The figure shows three views and two pictorial views of one solid part (mm, origin at its lowest corner). Answer the questions. Give positions to 0.01 mm unless a question says otherwise; leave off trailing zeros. Write each loop counter-clockwise with the first axis right and the second up, starting at its lowest first coordinate (ties: lowest second). Pieces come first, ordered by that corner, then holes. Notation, with made-up numbers: (-23, 77) -> (30, 77) arc R27 cw to (30, 106) -> close; hole circle Ø5 at (-11, -29). An arc over 180 degrees is marked (long way). Use a Markdown table: item, result.
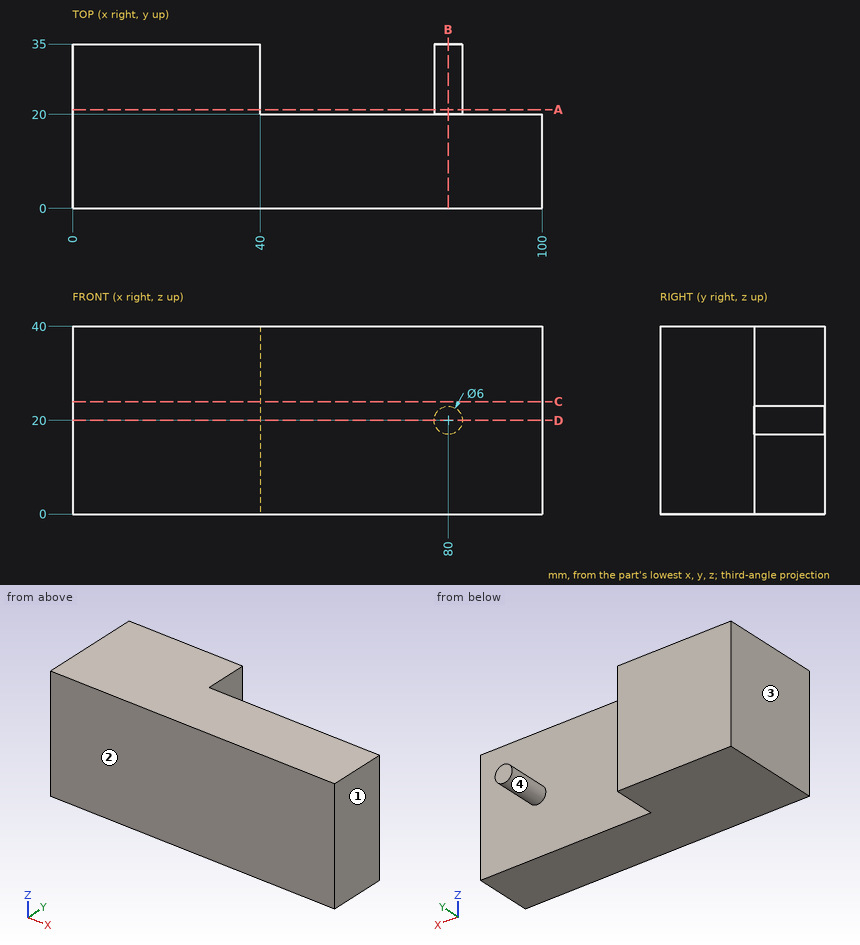
Item 1: A cutting plane is placed at B-B (x = 80). Give the vertices of the cut face in (y, z).
Return value:
| item | result |
|---|---|
| outline | (0, 0) -> (20, 0) -> (20, 17) -> (35, 17) -> (35, 23) -> (20, 23) -> (20, 40) -> (0, 40) -> close |
Item 2: Straight lines are drawn through the part: line 1 along X through (y, z) = (31, 38); line 2 along Y through (x, z) = (49.5, 17). For each, find the intervals that lie inside material, in ascending order. Write a range as [from, to].
Return value:
| item | result |
|---|---|
| line 1 | [0, 40] |
| line 2 | [0, 20] |
Item 3: A cutting plane is placed at A-A (y = 21). Give the vertices of the cut face in (x, z).
Return value:
| item | result |
|---|---|
| outline | (0, 0) -> (40, 0) -> (40, 40) -> (0, 40) -> close; circle Ø6 at (80, 20) |
Item 4: A cutting plane is placed at D-D (z = 20). Give the vertices of the cut face in (x, y).
Return value:
| item | result |
|---|---|
| outline | (0, 0) -> (100, 0) -> (100, 20) -> (83, 20) -> (83, 35) -> (77, 35) -> (77, 20) -> (40, 20) -> (40, 35) -> (0, 35) -> close |
Item 5: A cutting plane is placed at C-C (z = 24). Give the vertices of the cut face in (x, y).
Return value:
| item | result |
|---|---|
| outline | (0, 0) -> (100, 0) -> (100, 20) -> (40, 20) -> (40, 35) -> (0, 35) -> close |
Item 6: Each of these flat-tipped pins is pushed along its axis until it touches: P1, Ø5, axis at y = 31, z = 36, coming from the +X side; P2, Ø1.5, axis at x = 79, y = 13, coming from the -Z side; P3, Ø20, axis at x = 62, z = 25, coming from the +Y side; P4, Ø12, axis at y = 27, z = 24, coming from the +X side. Where does it stop, or does it pass through?
Return value:
| item | result |
|---|---|
| P1 | x = 40 |
| P2 | z = 0 |
| P3 | y = 20 |
| P4 | x = 83 |
Item 7: For a pull along X with two mould halves and no side action, classify the marked faces 1, 2, 3 and 4 as +X half, -X half, draft (parallel to the pull), parting line (faces both ways), or undercut.
Return value:
| item | result |
|---|---|
| face 1 | +X half |
| face 2 | draft |
| face 3 | -X half |
| face 4 | undercut |
